Work out the finished part from the listing and answer in its coordinate system (mm). A direction names the side the tool comes from. Give positions to 0.01 mm unless a question says otherwise; leave off trailing zeros. Order: outer loops, then holes, each group sorted by start corner. A loop starts at its lowest first (then second) coordinate and runs counter-clockwise, first axis right, second up. Notation, with made-up numbers: (46.25, -23) -> (91.25, -23) arc R24 ccw to (91.25, 2) -> close; hole circle Ø7 at (-2, -31). An arc over 180 degrees is marked (long way). Use a Markdown table: item, result. Add a question column.
```python
from build123d import *

# Parameters (mm, degrees)
SKETCH1_R           = 3.95
BOSS_EXTRUDE1_DEPTH = 110
SKETCH2_R           = 6.95
BOSS_EXTRUDE2_DEPTH = 1
CHAMFER1_SIZE       = 3
FILLET1_R           = 8


with BuildPart() as part:
    # Sketch1 → Boss-Extrude1 (new body)
    with BuildSketch(Plane(origin=(0, 0, 0), x_dir=(1, 0, 0), z_dir=(0, 1, 0))):
        with Locations(Location((0, 0, 0), (0, 0, 270))):
            Circle(SKETCH1_R)
    extrude(amount=BOSS_EXTRUDE1_DEPTH)

    # Sketch2 → Boss-Extrude2 (add)
    with BuildSketch(Plane(origin=(0, 39, 0), x_dir=(-1, 0, 0), z_dir=(0, -1, 0))):
        with Locations(Location((0, 0, 0), (0, 0, 90))):
            Circle(SKETCH2_R)
    extrude(amount=-BOSS_EXTRUDE2_DEPTH)

    # Chamfer1
    chamfer1_edges = [part.edges().sort_by_distance(p)[0] for p in [
        (0, 39, -3.95),
    ]]
    chamfer(chamfer1_edges, length=CHAMFER1_SIZE - 0.0001)  # a hair under: the kernel refuses the full size

    # Fillet1
    fillet1_edges = [part.edges().sort_by_distance(p)[0] for p in [
        (0, 36.0001, -3.95),
    ]]
    fillet(fillet1_edges, radius=FILLET1_R)


solid = part.part
```
1) Flat-ended cylindrical pins translate along their axes: pin 1 (1.5 mm diameter, centred on y = 91.5, z = 2.5, fed in from +X); pin 2 (1 mm diameter, centred on x = 3.5, y = 95.5, fed in from -Z); pin 3 (4 mm diameter, centred on y = 75.5, z = 3.5, fed in from +X). Find the tip coordinate at first contact, or state that the pin passes through.
2) Which of the six approach directions +Z, -Z, +X, -X, +Y, -Y give full straight-line access (tool end or side, diameter ignored) to faces 1 (the cylindrical face through (-6.785, 39.493, 1.507)), 2 (the cylindrical face through (2.67, 74.51, -2.91)), 3 (the cylindrical face through (1.186, 16.114, 3.768))?
3) The part is cut by section A-A, the plane y = 64. Determine the outline of the cut face in (x, z), then the cut area to 3 significant figures.
4) Straight lines are drawn through the part: line 1 (Z direction, x = 0.25, y = 4); line 2 (X direction, y = 57, z = 0.75); line 3 (X direction, y = 19.5, z = 2.5). For each, find the intervals that lie inside material, in ascending order.
A:
| question | item | result |
|---|---|---|
| 1 | pin 1 | x = 3.54 |
| 1 | pin 2 | z = -2.57 |
| 1 | pin 3 | x = 3.65 |
| 2 | face 1 | +Y, -Y |
| 2 | face 2 | +Y |
| 2 | face 3 | -Y |
| 3 | outline | circle Ø7.9 at (0, 0) |
| 3 | area | 49.0 mm^2 |
| 4 | line 1 | -3.94 to 3.94 |
| 4 | line 2 | -3.88 to 3.88 |
| 4 | line 3 | -3.06 to 3.06 |
